Could you check a few things on this drawing? It's one solid part, dimensions in mm from its lowest x, y, z. Give positions to 0.01 mm unless a question says otherwise; leave off trailing zeros. Loops run counter-clockwise (first coordinate to the right, second up) from the corner with the lowest first, then second, coordinate; pieces in that order, holes last. Notation, with made-up numbers: (-39, 73.5) - (-3, 73.5) arc R12 cw to (-3, 79.5) - close; hole circle Ø7 at (-26, -38.75). An arc over 180 degrees is marked (long way). Write item = value, one per line.
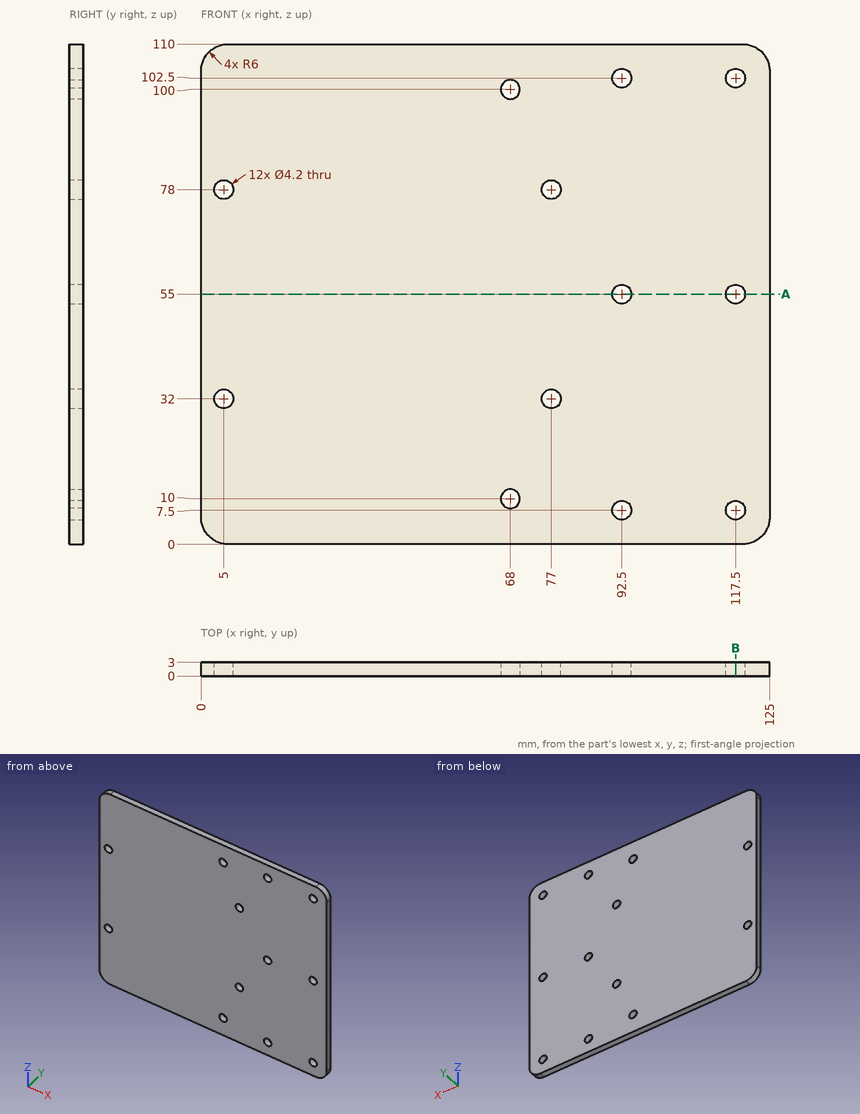
Q1. Imagine slicing it at B-B, the plane x = 117.5. Write out the boundary of the cut face in (y, z), then the cut area to 3 significant figures.
Output:
outline = (0, 0) - (3, 0) - (3, 5.4) - (0, 5.4) - close; (0, 9.6) - (3, 9.6) - (3, 52.9) - (0, 52.9) - close; (0, 57.1) - (3, 57.1) - (3, 100.4) - (0, 100.4) - close; (0, 104.6) - (3, 104.6) - (3, 110) - (0, 110) - close
area = 292 mm2
Q2. Imagine slicing it at A-A, the plane z = 55. Write out the boundary of the cut face in (x, y), then the cut area to 3 significant figures.
Output:
outline = (0, 0) - (90.4, 0) - (90.4, 3) - (0, 3) - close; (94.6, 0) - (115.4, 0) - (115.4, 3) - (94.6, 3) - close; (119.6, 0) - (125, 0) - (125, 3) - (119.6, 3) - close
area = 350 mm2
Q3. I need wall thicknesses on L1, parallel to X at y = 2.1, z = 7.5; L2, parallel to X at y = 1.05, z = 32; L3, parallel to Z at x = 93, y = 0.3. Which ranges of each line are inside material? Lowest first, please.
Output:
L1 = 0 to 90.4, 94.6 to 115.4, 119.6 to 125
L2 = 0 to 2.9, 7.1 to 74.9, 79.1 to 125
L3 = 0 to 5.46, 9.54 to 52.96, 57.04 to 100.46, 104.54 to 110
Q4. For pin 1 (5.5 mm diameter, centred on x = 5, z = 78, fed in from -Y), with a flat end and sliding along its axis, tell me the tip position at first contact or that it passes through.
Output:
pin_1 = 0
